```python
from build123d import *
from OCP.BRepFilletAPI import BRepFilletAPI_MakeChamfer

# Parameters (mm, degrees)
SKETCH1_W           = 80
SKETCH1_H           = 110
BOSS_EXTRUDE1_DEPTH = 3
SKETCH2_W           = 40.4
SKETCH2_H           = 3
CUT_EXTRUDE1_DEPTH  = 15
FILLET1_R           = 4
SKETCH7_W           = 73.6
SKETCH7_H           = 86.6
BOSS_EXTRUDE2_DEPTH = 2
SKETCH3_R           = 12.7
CUT_EXTRUDE2_DEPTH  = 69.190908485
SKETCH4_R           = 6
SKETCH4_R_2         = 3.2
SKETCH4_R_3         = 3.7
SKETCH4_R_4         = 1.6
CUT_EXTRUDE3_DEPTH  = 69.190908485
CHAMFER2_SIZE       = 1.5
CHAMFER2_SIZE2      = 0.545955351
CHAMFER3_SIZE       = 2.309401077
CHAMFER3_SIZE_2     = 4
BOSS_EXTRUDE3_DEPTH = 1
CHAMFER4_SIZE       = 1
CHAMFER4_SIZE2      = 0.363970234
CUT_EXTRUDE4_DEPTH  = 4
CUT_EXTRUDE5_START  = -4
CUT_EXTRUDE5_DEPTH  = 4


with BuildPart() as part:
    # Sketch1 → Boss-Extrude1 (new body)
    with BuildSketch(Plane(origin=(0, 0, 0), x_dir=(1, 0, 0), z_dir=(0, 1, 0))):
        Rectangle(SKETCH1_W, SKETCH1_H)
    extrude(amount=BOSS_EXTRUDE1_DEPTH)

    # Sketch2 → Cut-Extrude1 (cut)
    with BuildSketch(Plane.XY.offset(55)):
        with Locations((0, 1.5)):
            Rectangle(SKETCH2_W, SKETCH2_H)
    extrude(amount=-CUT_EXTRUDE1_DEPTH, mode=Mode.SUBTRACT)

    # Fillet1
    fillet1_edges = [part.edges().sort_by_distance(p)[0] for p in [
        (-20.2, 1.5, 55),
        (20.2, 1.5, 55),
        (40, 1.5, 55),
        (-40, 1.5, 55),
    ]]
    fillet(fillet1_edges, radius=FILLET1_R)

    # Sketch7 → Boss-Extrude2 (add)
    with BuildSketch(Plane.XZ):
        with Locations((0, -8.5)):
            Rectangle(SKETCH7_W, SKETCH7_H)
    extrude(amount=BOSS_EXTRUDE2_DEPTH)

    # Sketch3 → Cut-Extrude2 (cut, through all)
    with BuildSketch(Plane(origin=(0, 3, 0), x_dir=(1, 0, 0), z_dir=(0, 1, 0))):
        with Locations(Location((-22, 0, 0), (0, 0, 270))):
            Circle(SKETCH3_R)
        with Locations(Location((10, -10, 0), (0, 0, 270))):
            Circle(SKETCH3_R)
    extrude(amount=-CUT_EXTRUDE2_DEPTH, mode=Mode.SUBTRACT)

    # Sketch4 → Cut-Extrude3 (cut, through all)
    with BuildSketch(Plane(origin=(0, 3, 0), x_dir=(1, 0, 0), z_dir=(0, 1, 0))):
        with Locations(Location((19, 23, 0), (0, 0, 270))):
            Circle(SKETCH4_R)
        with Locations(Location((-22, 23, 0), (0, 0, 270))):
            Circle(SKETCH4_R_2)
        with Locations(Location((31, -10, 0), (0, 0, 270))):
            Circle(SKETCH4_R_2)
        with Locations(Location((30.1, -41, 0), (0, 0, 270))):
            Circle(SKETCH4_R_3)
        with Locations(Location((-29, 40, 0), (0, 0, 270))):
            Circle(SKETCH4_R_2)
        with Locations(Location((-15, 40, 0), (0, 0, 270))):
            Circle(SKETCH4_R_2)
        with Locations(Location((27, 40, 0), (0, 0, 270))):
            Circle(SKETCH4_R_2)
        with Locations(Location((-22, -25, 0), (0, 0, 270))):
            Circle(SKETCH4_R_2)
        with Locations(Location((-30, -47, 0), (0, 0, 270))):
            Circle(SKETCH4_R_4)
        with Locations(Location((-34, 49, 0), (0, 0, 270))):
            Circle(SKETCH4_R_4)
        with Locations(Location((34, 49, 0), (0, 0, 270))):
            Circle(SKETCH4_R_4)
        with Locations(Location((32, -49, 0), (0, 0, 270))):
            Circle(SKETCH4_R_4)
    extrude(amount=-CUT_EXTRUDE3_DEPTH, mode=Mode.SUBTRACT)

    # Chamfer2: one chamfer whose edges measure the first distance from different faces: ONE call of the kernel's chamfer builder (chamfer() names one face for all edges)
    chamfer2_edges_1 = [part.edges().sort_by_distance(p)[0] for p in [
        (-36.8, -2, -8.5),
    ]]
    chamfer2_side_1 = [part.faces().sort_by_distance(p)[0] for p in [
        (-36.8, -1, -8.5),
    ]]
    chamfer2_edges_2 = [part.edges().sort_by_distance(p)[0] for p in [
        (0, -2, -51.8),
    ]]
    chamfer2_side_2 = [part.faces().sort_by_distance(p)[0] for p in [
        (0, -1, -51.8),
    ]]
    chamfer2_edges_3 = [part.edges().sort_by_distance(p)[0] for p in [
        (36.8, -2, -8.5),
    ]]
    chamfer2_side_3 = [part.faces().sort_by_distance(p)[0] for p in [
        (36.8, -1, -8.5),
    ]]
    chamfer2_edges_4 = [part.edges().sort_by_distance(p)[0] for p in [
        (0, -2, 34.8),
    ]]
    chamfer2_side_4 = [part.faces().sort_by_distance(p)[0] for p in [
        (0, -1, 34.8),
    ]]
    chamfer2 = BRepFilletAPI_MakeChamfer(part.part.solid().wrapped)
    for e in chamfer2_edges_1:
        chamfer2.Add(CHAMFER2_SIZE, CHAMFER2_SIZE2, e.wrapped, chamfer2_side_1[0].wrapped)  # the first distance lies on this face
    for e in chamfer2_edges_2:
        chamfer2.Add(CHAMFER2_SIZE, CHAMFER2_SIZE2, e.wrapped, chamfer2_side_2[0].wrapped)  # the first distance lies on this face
    for e in chamfer2_edges_3:
        chamfer2.Add(CHAMFER2_SIZE, CHAMFER2_SIZE2, e.wrapped, chamfer2_side_3[0].wrapped)  # the first distance lies on this face
    for e in chamfer2_edges_4:
        chamfer2.Add(CHAMFER2_SIZE, CHAMFER2_SIZE2, e.wrapped, chamfer2_side_4[0].wrapped)  # the first distance lies on this face
    add(Compound.cast(chamfer2.Shape()), mode=Mode.REPLACE)

    # Chamfer3
    # the kernel refuses this chamfer: 4, 2.309401077 mm, written as the material it takes off along each edge
    with BuildSketch(Plane(origin=(-22, -2, 0), x_dir=(0, 0, 1), z_dir=(-1, 0, 0))) as chamfer3_piece_1:
        Polygon((12.7 + CHAMFER3_SIZE, 0), (12.7, CHAMFER3_SIZE_2), (12.7, 0), align=None)
    revolve(axis=Axis((-22, -2, 0), (0, 1, 0)), mode=Mode.SUBTRACT)
    with BuildSketch(Plane(origin=(10, -2, 10), x_dir=(0, 0, 1), z_dir=(-1, 0, 0))) as chamfer3_piece_2:
        Polygon((12.7 + CHAMFER3_SIZE, 0), (12.7, CHAMFER3_SIZE_2), (12.7, 0), align=None)
    revolve(axis=Axis((10, -2, 10), (0, 1, 0)), mode=Mode.SUBTRACT)

    # Sketch8 → Boss-Extrude3 (add)
    with BuildSketch(Plane(origin=(0, 3, 0), x_dir=(1, 0, 0), z_dir=(0, 1, 0))):
        Polygon((-35, 43), (-35, 46), (-9, 46), (-9, 43), (-10, 43), (-10, 45), (-34, 45), (-34, 43), align=None)
        Polygon((-9, 37), (-9, 34), (-35, 34), (-35, 37), (-34, 37), (-34, 35), (-10, 35), (-10, 37), align=None)
        Polygon((-37, 12), (-37, 15), (-7, 15), (-7, 12), (-8, 12), (-8, 14), (-36, 14), (-36, 12), align=None)
        Polygon((-4.5, 10), (-4.5, 13), (35.5, 13), (35.5, 10), (34.5, 10), (34.5, 12), (-3.5, 12), (-3.5, 10), align=None)
        Polygon((-7, -12), (-7, -15), (-37, -15), (-37, -12), (-36, -12), (-36, -14), (-8, -14), (-8, -12), align=None)
        Polygon((-37, -19.5), (-37, -16.5), (-7, -16.5), (-7, -19.5), (-8, -19.5), (-8, -17.5), (-36, -17.5), (-36, -19.5), align=None)
        Polygon((-7, -30.5), (-7, -33.5), (-37, -33.5), (-37, -30.5), (-36, -30.5), (-36, -32.5), (-8, -32.5), (-8, -30.5), align=None)
    extrude(amount=BOSS_EXTRUDE3_DEPTH)

    # Chamfer4: one chamfer whose edges measure the first distance from different faces: ONE call of the kernel's chamfer builder (chamfer() names one face for all edges)
    chamfer4_edges_1 = [part.edges().sort_by_distance(p)[0] for p in [
        (-22, -2, 21.8),
    ]]
    chamfer4_side_1 = [part.faces().sort_by_distance(p)[0] for p in [
        (-22, 0.5, 21.8),
    ]]
    chamfer4_edges_2 = [part.edges().sort_by_distance(p)[0] for p in [
        (-22, -2, -26.2),
    ]]
    chamfer4_side_2 = [part.faces().sort_by_distance(p)[0] for p in [
        (-22, 0.5, -26.2),
    ]]
    chamfer4_edges_3 = [part.edges().sort_by_distance(p)[0] for p in [
        (31, -2, 6.8),
    ]]
    chamfer4_side_3 = [part.faces().sort_by_distance(p)[0] for p in [
        (31, 0.5, 6.8),
    ]]
    chamfer4_edges_4 = [part.edges().sort_by_distance(p)[0] for p in [
        (30.1, 0, 37.3),
    ]]
    chamfer4_side_4 = [part.faces().sort_by_distance(p)[0] for p in [
        (30.1, 1.5, 37.3),
    ]]
    chamfer4_edges_5 = [part.edges().sort_by_distance(p)[0] for p in [
        (-29, -2, -43.2),
    ]]
    chamfer4_side_5 = [part.faces().sort_by_distance(p)[0] for p in [
        (-29, 0.5, -43.2),
    ]]
    chamfer4_edges_6 = [part.edges().sort_by_distance(p)[0] for p in [
        (-15, -2, -43.2),
    ]]
    chamfer4_side_6 = [part.faces().sort_by_distance(p)[0] for p in [
        (-15, 0.5, -43.2),
    ]]
    chamfer4_edges_7 = [part.edges().sort_by_distance(p)[0] for p in [
        (19, -2, -29),
    ]]
    chamfer4_side_7 = [part.faces().sort_by_distance(p)[0] for p in [
        (19, 0.5, -29),
    ]]
    chamfer4_edges_8 = [part.edges().sort_by_distance(p)[0] for p in [
        (27, -2, -43.2),
    ]]
    chamfer4_side_8 = [part.faces().sort_by_distance(p)[0] for p in [
        (27, 0.5, -43.2),
    ]]
    chamfer4 = BRepFilletAPI_MakeChamfer(part.part.solid().wrapped)
    for e in chamfer4_edges_1:
        chamfer4.Add(CHAMFER4_SIZE, CHAMFER4_SIZE2, e.wrapped, chamfer4_side_1[0].wrapped)  # the first distance lies on this face
    for e in chamfer4_edges_2:
        chamfer4.Add(CHAMFER4_SIZE, CHAMFER4_SIZE2, e.wrapped, chamfer4_side_2[0].wrapped)  # the first distance lies on this face
    for e in chamfer4_edges_3:
        chamfer4.Add(CHAMFER4_SIZE, CHAMFER4_SIZE2, e.wrapped, chamfer4_side_3[0].wrapped)  # the first distance lies on this face
    for e in chamfer4_edges_4:
        chamfer4.Add(CHAMFER4_SIZE, CHAMFER4_SIZE2, e.wrapped, chamfer4_side_4[0].wrapped)  # the first distance lies on this face
    for e in chamfer4_edges_5:
        chamfer4.Add(CHAMFER4_SIZE, CHAMFER4_SIZE2, e.wrapped, chamfer4_side_5[0].wrapped)  # the first distance lies on this face
    for e in chamfer4_edges_6:
        chamfer4.Add(CHAMFER4_SIZE, CHAMFER4_SIZE2, e.wrapped, chamfer4_side_6[0].wrapped)  # the first distance lies on this face
    for e in chamfer4_edges_7:
        chamfer4.Add(CHAMFER4_SIZE, CHAMFER4_SIZE2, e.wrapped, chamfer4_side_7[0].wrapped)  # the first distance lies on this face
    for e in chamfer4_edges_8:
        chamfer4.Add(CHAMFER4_SIZE, CHAMFER4_SIZE2, e.wrapped, chamfer4_side_8[0].wrapped)  # the first distance lies on this face
    add(Compound.cast(chamfer4.Shape()), mode=Mode.REPLACE)

    # Sketch9 → Cut-Extrude4 (cut)
    with BuildSketch(Plane(origin=(36.8, 0, 0), x_dir=(0, 0, -1), z_dir=(1, 0, 0))):
        with BuildLine():
            Line((40.46, -2), (32.46, -2))
            ThreePointArc((32.46, -2), (36.46, -0.5), (40.46, -2))
        make_face()
    extrude(amount=-CUT_EXTRUDE4_DEPTH, mode=Mode.SUBTRACT)

    # Sketch10 → Cut-Extrude5 (cut)
    with BuildSketch(Plane.ZY.offset(36.8).offset(CUT_EXTRUDE5_START)):
        with BuildLine():
            Line((-40.46, -2), (-32.46, -2))
            ThreePointArc((-32.46, -2), (-36.46, -0.5), (-40.46, -2))
        make_face()
    extrude(amount=CUT_EXTRUDE5_DEPTH, mode=Mode.SUBTRACT)


solid = part.part
```
CAD build for the part. Positions are in the model's coordinates, mm. A direction names the side the tool comes from. Round coordinates to 2 decimals unless told otherwise and drop trailing zeros. Return JSON: item names as keys, results as strings. Group by question number.
Q1. Tool access for faces 4 (the face through (34.8, -0.5, -36.4)), 5 (the face through (21.403, 1.521, 53.859)), 6 (the face through (31.39, 1.52, 50.48)): list every direction of +Z, -Z, +X, -X, +Y, -Y with a clear straight run to the whole face (end or side of a thin tool).
Q2. Band-saw the part on A-A on z = 41.5. Give the number of separate pieces and of enclosed holes in the cut face, plus the area to 3 significant figures.
Q3. Drill centre lines: line 1 along X through (y, z) = (-0.1, -40); line 2 along X through (y, z) = (2, 49); line 3 along X through (y, z) = (2.2, -40). Where is each one in solid material? Low to high. Write a range as [from, to].
Q4. Two-plate mould, pull along Z, no slides. Class faces 1 (the face through (34.173, 1.028, 9.583)), 2 (the face through (-20.2, 1, 46)), 3 (the face through (-30, 1, 55)): +Z half, -Z half, draft (parallel to the pull), parting line (faces both ways), or undercut.
Q5. Flat gauge pins, fed straight in: pin 1 Ø3.5 at (x, z) = (32, 49) entering from +Y; pin 2 Ø1.1 at (x, y) = (-36.5, 3.5) entering from +Z; pin 3 Ø0.5 at (y, z) = (3.5, 13.5) entering from +X. Where does each tip first touch, or does it go through?
Solutions:
{
 "1": {"face 4": "+X, -Y", "face 5": "+Z, +Y, -Y", "face 6": "+Y, -Y"},
 "2": {"separate pieces": "3", "enclosed holes": "0", "area": "96.4 mm^2"},
 "3": {"line 1": "x = [-36.8, -32.2], [-25.8, -18.2], [-11.8, 23.8], [30.2, 36.8]", "line 2": "x = [-40, -20.2], [20.2, 30.4], [33.6, 40]", "line 3": "x = [-40, -32.2], [-25.8, -18.2], [-11.8, 23.8], [30.2, 40]"},
 "4": {"face 1": "undercut", "face 2": "draft", "face 3": "+Z half"},
 "5": {"pin 1": "stops at y = 3", "pin 2": "stops at z = 54.99", "pin 3": "stops at x = -7"}
}
